For this review, take the finished solid that the model builds, in its own axes (mm). Face numbers are marked on the shaded views. A direction names the side the tool comes from. Coordinates: 2 decimals unless noted, no trailing zeros. Loops run counter-clockwise (first coordinate to the right, second up) from the corner with the lowest first, then second, coordinate; pieces in that order, holes last. Notation, with made-up numbers: (69, 13) - (120, 13) arc R7 cw to (120, 21) - close; hole circle Ø11 at (-9.5, 35.25). An arc over 180 degrees is marked (long way). One line per item, written item: value. Start each with the question number.
1. For the marked faces 4, 5, 6 and 7, list the 3-axis set-ups (+Z, -Z, +X, -X, +Y, -Y) from which the entire face can be reached by the end or side of a thin tool; tool diameter is ignored.
2. Take a section at B-B, the plane x = 0. State the section outline as (y, z) points (3 decimals).
3. To check wall thickness, follow line 1 (Y direction, x = 20, z = 40); line 2 (Z direction, x = -30.5, y = 16) (3 decimals); line 3 (X direction, y = -10.5, z = 40). State the ranges of each line that lie inside material, in increasing order. Write a range as from..to.
4. The part is to be moulded in two halves that separate along Y. For the marked faces 1, 2 and 3, say which applies: released by +Y, released by -Y, zero draft, split by the parting line, or undercut.
5. Insertion check: pin 1 (10 mm diameter, centred on y = 33, z = 31.5, fed in from +X); pin 2 (2 mm diameter, centred on x = -11.5, y = 32, fed in from -Z); pin 3 (12.5 mm diameter, centred on x = 46, z = 39, fed in from +Y). Each pin has a flat end and moves straight along its axis. Give the tip position at first contact, or say it passes through.
6. Take a section at A-A, the plane y = 8. State the section outline as (x, z) points (3 decimals), and give its area (3 significant figures).
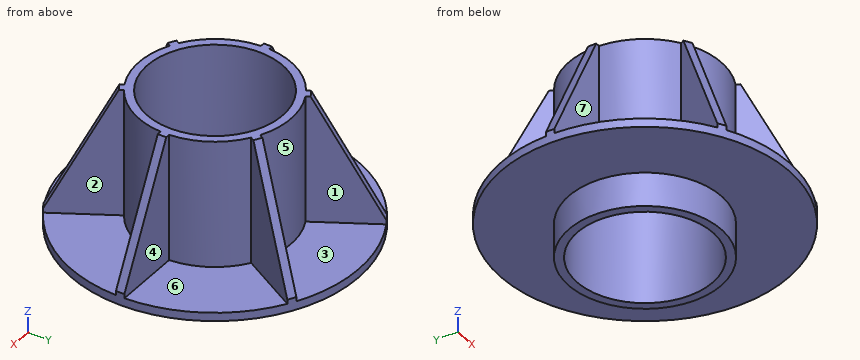
```python
from build123d import *

# Parameters (mm, degrees)
F0_R            = 28.575
F0_R_2          = 25.4
F1_DEPTH        = 12.7
F2_R            = 53.975
F2_R_2          = 25.4
F3_DEPTH        = 50.8
F6_DEPTH        = 47.625
F6_COPIES_COUNT = 6


# Not quite as in the source:
# - a pattern or mirror of a feature is missing from the dataset's text; its kind, count and spacing are read off the source's solid


with BuildPart() as f1:
    # F0 (on Top) → F1 (new body)
    with BuildSketch(Plane.XY):
        Circle(F0_R)
        Circle(F0_R_2, mode=Mode.SUBTRACT)
    extrude(amount=F1_DEPTH)

    # F2 (on face) → F3 (join)
    with BuildSketch(Plane.XY.offset(12.7)):
        Circle(F2_R)
        Circle(F2_R_2, mode=Mode.SUBTRACT)
    extrude(amount=F3_DEPTH)

    # F5 (on face) → F6 (cut, through all)
    with BuildSketch(Plane.XY.offset(63.5)):
        with BuildLine():
            ThreePointArc((-15.6402496783, -23.9147070858), (-24.7466759131, -14.2875), (-28.5308686995, -1.5875))
            Line((-28.5308686995, -1.5875), (-53.9516493608, -1.5875))
            ThreePointArc((-53.9516493608, -1.5875), (-46.7437211693, -26.9875), (-28.3506400089, -45.9297489225))
            Line((-28.3506400089, -45.9297489225), (-15.6402496783, -23.9147070858))
        make_face()
    f6 = extrude(amount=-F6_DEPTH, mode=Mode.SUBTRACT)

    # F6_copies: F6 ×6 about axis
    f6_copies_axis = Axis((0, 0, 0), (0, 0, 1))
    for i in range(1, F6_COPIES_COUNT):
        add(f6.rotate(f6_copies_axis, i * 360 / F6_COPIES_COUNT), mode=Mode.SUBTRACT)

    # F7 (on Front) → F8 (revolve, cut)
    with BuildSketch(Plane.XZ):
        Polygon((-53.975, 17.4625), (-30.1625, 63.5), (-53.975, 63.5), align=None)
    revolve(axis=Axis((0, 0, 0), (0, 0, -1)), mode=Mode.SUBTRACT)


solid = f1.part
```
Solutions:
1. face 4: +Z, +X, +Y
1. face 5: +Z, +Y
1. face 6: +Z, +X
1. face 7: +Z, -X, -Y
2. outline: (-53.975, 12.7) - (-28.575, 12.7) - (-28.575, 0) - (-25.4, 0) - (-25.4, 63.5) - (-28.575, 63.5) - (-28.575, 15.875) - (-53.975, 15.875) - close; (25.4, 0) - (28.575, 0) - (28.575, 12.7) - (53.975, 12.7) - (53.975, 15.875) - (28.575, 15.875) - (28.575, 63.5) - (25.4, 63.5) - close
3. line 1: -37.29..-31.47, -20.41..-15.66, 15.66..20.41, 31.47..37.29
3. line 2: 12.7..15.875
3. line 3: -26.58..-23.13, 23.13..26.58
4. face 1: released by +Y
4. face 2: undercut
4. face 3: zero draft
5. pin 1: x = 23.77
5. pin 2: z = 12.7
5. pin 3: y = 1.59
6. outline: (-53.379, 12.7) - (-27.432, 12.7) - (-27.432, 0) - (-24.107, 0) - (-24.107, 63.5) - (-27.432, 63.5) - (-27.432, 15.875) - (-53.379, 15.875) - close; (24.107, 0) - (27.432, 0) - (27.432, 12.7) - (53.379, 12.7) - (53.379, 15.875) - (27.432, 15.875) - (27.432, 63.5) - (24.107, 63.5) - close
6. area: 587 mm2
